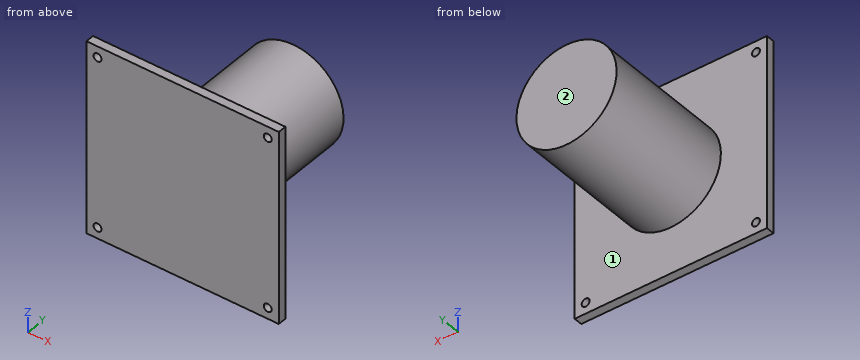
from build123d import *

# Parameters (mm, degrees)
SKETCH_1_W          = 38.4
SKETCH_1_H          = 38.4
EXTRUDE_1_DEPTH     = 1.7
SKETCH_2_R          = 10
EXTRUDE_2_DEPTH     = 27
SKETCH_3_R          = 0.8
CUT_EXTRUDE_1_DEPTH = 10


with BuildPart() as part:
    # 草图1 → 凸台-拉伸1 (new body)
    with BuildSketch(Plane(origin=(0, 0, 0), x_dir=(1, 0, 0), z_dir=(0, 1, 0))):
        Rectangle(SKETCH_1_W, SKETCH_1_H)
    extrude(amount=EXTRUDE_1_DEPTH)

    # 草图2 → 凸台-拉伸2 (add)
    with BuildSketch(Plane(origin=(0, 1.7, 0), x_dir=(1, 0, 0), z_dir=(0, 1, 0))):
        with Locations(Location((0, 0, 0), (0, 0, 270))):
            Circle(SKETCH_2_R)
    extrude(amount=EXTRUDE_2_DEPTH)

    # 草图3 → 切除-拉伸1 (cut)
    with BuildSketch(Plane.XZ):
        with Locations(Location((-17, 17, 0), (0, 0, 270))):
            Circle(SKETCH_3_R)
        with Locations(Location((17, 17, 0), (0, 0, 270))):
            Circle(SKETCH_3_R)
        with Locations(Location((17, -17, 0), (0, 0, 270))):
            Circle(SKETCH_3_R)
        with Locations(Location((-17, -17, 0), (0, 0, 270))):
            Circle(SKETCH_3_R)
    extrude(amount=-CUT_EXTRUDE_1_DEPTH, mode=Mode.SUBTRACT)


solid = part.part
Read the model definition and answer for the solid it produces. Units are mm, in the model's axes. Face numbers are marked on the shaded views. A direction names the side the tool comes from. Coordinates: 2 decimals unless noted, no trailing zeros. Loops run counter-clockwise (first coordinate to the right, second up) from the corner with the lowest first, then second, coordinate; pieces in that order, holes last. Notation, with made-up numbers: (27, 68) -> (42, 68) arc R33 cw to (42, 105) -> close; hole circle Ø4 at (-29.5, 55.25). An arc over 180 degrees is marked (long way). Answer in a Markdown table with one row per item.
Item 1: A cutting plane is placed at C-C on z = 3.5. Determine the outline of the cut face in (x, y).
Returned:
| item | result |
|---|---|
| outline | (-19.2, 0) -> (19.2, 0) -> (19.2, 1.7) -> (9.37, 1.7) -> (9.37, 28.7) -> (-9.37, 28.7) -> (-9.37, 1.7) -> (-19.2, 1.7) -> close |
Item 2: Each of these flat-tipped pins is pushed along its axis until it touches: P1, Ø12, axis at y = 16, z = 1.5, coming from the +X side; P2, Ø2, axis at x = -17, z = -17, coming from the +Y side; P3, Ø2, axis at y = 25.5, z = -5, coming from the +X side; P4, Ø1.3, axis at x = 17, z = 17, coming from the -Y side. Where does it stop, or does it pass through?
Returned:
| item | result |
|---|---|
| P1 | stops at x = 10 |
| P2 | stops at y = 1.7 |
| P3 | stops at x = 9.17 |
| P4 | passes through |
Item 3: For the marked faces 1 and 2, determine the directions among +Z, -Z, +X, -X, +Y, -Y from which every point of the face is accessible in a straight line to the end or side of a thin tool.
Returned:
| item | result |
|---|---|
| face 1 | +Y |
| face 2 | +Z, -Z, +X, -X, +Y |
Item 4: A cutting plane is placed at B-B on x = 0. Determine the outline of the cut face in (y, z), plus the area to 3 significant figures.
Returned:
| item | result |
|---|---|
| outline | (0, -19.2) -> (1.7, -19.2) -> (1.7, -10) -> (28.7, -10) -> (28.7, 10) -> (1.7, 10) -> (1.7, 19.2) -> (0, 19.2) -> close |
| area | 605 mm^2 |
Item 5: A cutting plane is placed at D-D on y = 23.5. Determine the outline of the cut face in (x, z).
Returned:
| item | result |
|---|---|
| outline | circle Ø20 at (0, 0) |
Item 6: A cutting plane is placed at A-A on x = -17. Determine the outline of the cut face in (y, z), plus the area to 3 significant figures.
Returned:
| item | result |
|---|---|
| outline | (0, -19.2) -> (1.7, -19.2) -> (1.7, -17.8) -> (0, -17.8) -> close; (0, -16.2) -> (1.7, -16.2) -> (1.7, 16.2) -> (0, 16.2) -> close; (0, 17.8) -> (1.7, 17.8) -> (1.7, 19.2) -> (0, 19.2) -> close |
| area | 59.8 mm^2 |
Item 7: Straight lines are drawn through the part: line 1 along X through (y, z) = (0.85, -17); line 2 along Y through (x, z) = (-12, -15); line 3 along X through (y, z) = (5, -6). For each, find the intervals that lie inside material, in ascending order. Write a range as [from, to].
Returned:
| item | result |
|---|---|
| line 1 | x = [-19.2, -17.8], [-16.2, 16.2], [17.8, 19.2] |
| line 2 | y = [0, 1.7] |
| line 3 | x = [-8, 8] |
